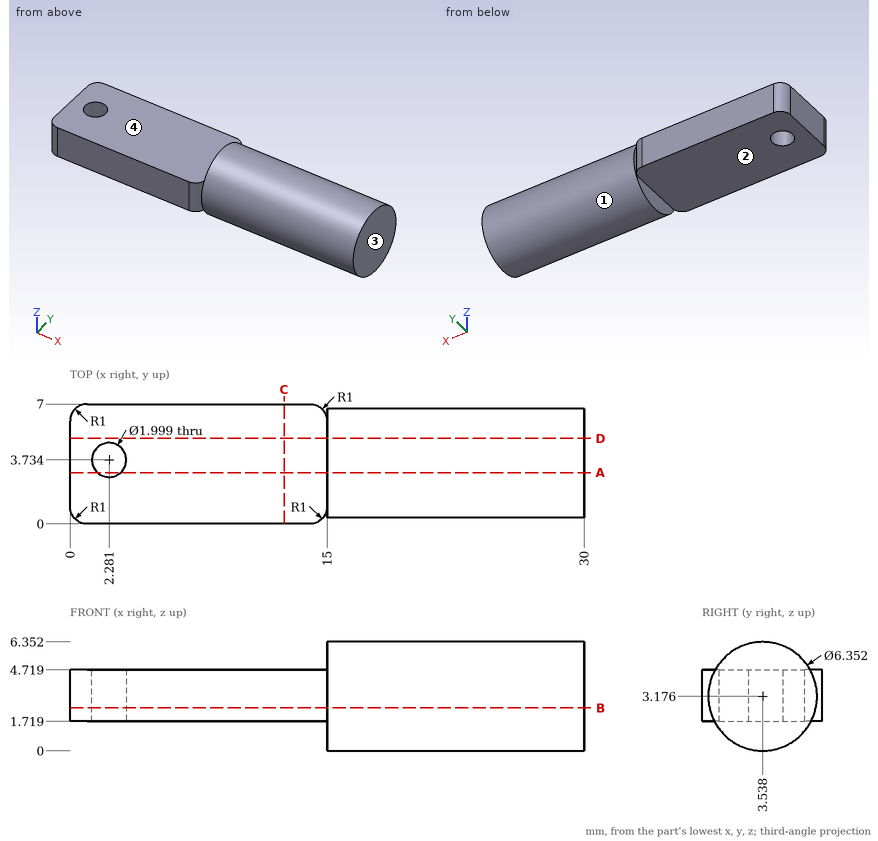
Job drawing, mm, ordinate dimensions from the low corner. One solid piece. A direction names the side the tool comes from. Coordinates: 2 decimals unless noted, no trailing zeros. Loops run counter-clockwise (first coordinate to the right, second up) from the corner with the lowest first, then second, coordinate; pieces in that order, holes last. Notation, with made-up numbers: (68.5, 66.25) -> (105.5, 66.25) arc R12 ccw to (105.5, 84.25) -> close; hole circle Ø1 at (65, -9). An arc over 180 degrees is marked (long way). One line per item, written item: value.
1. Slice it at C-C on x = 12.5. Write the cut outline in (y, z).
Answers:
outline: (0, 1.72) -> (7, 1.72) -> (7, 4.72) -> (0, 4.72) -> close
2. Which spindle directions (+Z, -Z, +X, -X, +Y, -Y) get a long thin tool onto all of the face, cutting with end or side? Do the marked faces 1, 2, 3 and 4. Say none if no direction does.
Answers:
face 1: +X
face 2: -Z, -X, +Y, -Y
face 3: +Z, -Z, +X, +Y, -Y
face 4: +Z, -X, +Y, -Y
3. Slice it at A-A on y = 3. Write the cut outline in (x, z) (1 decimal).
Answers:
outline: (0, 1.7) -> (1.6, 1.7) -> (1.6, 4.7) -> (0, 4.7) -> close; (3, 1.7) -> (15, 1.7) -> (15, 0) -> (30, 0) -> (30, 6.3) -> (15, 6.3) -> (15, 4.7) -> (3, 4.7) -> close
4. Slice it at B-B on z = 2.5. Write the cut outline in (x, y) (1 decimal).
Answers:
outline: (0, 1) arc R1 ccw to (1, 0) -> (14, 0) arc R1 ccw to (15, 1) -> (15, 0.4) -> (30, 0.4) -> (30, 6.6) -> (15, 6.6) -> (15, 6) arc R1 ccw to (14, 7) -> (1, 7) arc R1 ccw to (0, 6) -> close; hole circle Ø2 at (2.3, 3.7)
5. Drill centre lines: line 1 (X direction, y = 5.25, z = 1.25); line 2 (Z direction, x = 7, y = 6.25); line 3 (X direction, y = 4.25, z = 4.5) (1 decimal). Where is each one in solid material? Low to high. Write a range as [from, to].
Answers:
line 1: x = [15, 30]
line 2: z = [1.72, 4.72]
line 3: x = [0, 1.4], [3.1, 30]
6. Flat gauge pins, fed straight in: P1, Ø3.5, axis at x = 9, y = 2.5, coming from the +Z side; P2, Ø3, axis at x = 16, z = 3.5, coming from the +Y side (1 decimal); P3, Ø1, axis at x = 25.5, z = 1, coming from the +Y side (1 decimal). Where does each tip first touch, or does it go through?
Answers:
P1: stops at z = 4.72
P2: stops at y = 6.9
P3: stops at y = 6.2
7. Slice it at D-D on y = 5. Write the cut outline in (x, z) (1 decimal).
Answers:
outline: (0, 1.7) -> (15, 1.7) -> (15, 0.4) -> (30, 0.4) -> (30, 6) -> (15, 6) -> (15, 4.7) -> (0, 4.7) -> close
